Could you check a few things on this model? Use its own coordinates, in mm. Face numbers are marked on the shaded views. A direction names the side the tool comes from. Round coordinates to 2 decimals unless told otherwise and drop trailing zeros. Order: outer loops, then holes, each group sorted by start corner. A loop starts at its lowest first (then second) coordinate and runs counter-clockwise, first axis right, second up. Notation, with made-up numbers: (-25, 56) - (21, 56) arc R26 ccw to (21, 77) - close; hole circle Ø8 at (40, 44.5). An arc over 180 degrees is marked (long way). Return JSON: item names as keys, results as strings. Group by question number.
Autodesk Inventor part; units mm, degrees
ref_plane "Work Plane1" through (-3, -25.1, -19.1) normal (0, 0, 1) x (1, 0, 0)
ref_plane "YZ Plane" through (0, 0, 0) normal (1, 0, 0) x (0, 1, 0)
ref_plane "XZ Plane" through (0, 0, 0) normal (0, 1, 0) x (-1, 0, 0)
sketch "Sketch1" plane through (0, 0, 0) normal (1, 0, 0) x (0, 1, 0)
  line L0 (0, 0) -> (-25.1, 0)
  line L1 (-25.1, 0) -> (-25.1, -38.2)
  line L2 (-25.1, -38.2) -> (0, -38.2)
  line L3 (0, -38.2) -> (0, 0)
  circle A0 centre (-22.1, -15.85) radius 2.5
  circle A1 centre (-22.1, -22.35) radius 2.5
  arc A2 (-18.1, -15.85) -> (-25.1, -18.4958) centre (-22.1, -15.85) ccw
  arc A3 (-25.1, -19.7042) -> (-18.1, -22.35) centre (-22.1, -22.35) ccw
  line L4 (-18.1, -15.85) -> (-18.1, -22.35)
  line L5 (-22.1, -11.85) -> (-25.1, -11.85)
  line L6 (-22.1, -26.35) -> (-25.1, -26.35)
  line L7 (0, 0) -> (-25.1, 0)
  line L8 (-25.1, 0) -> (-25.1, 5)
  line L9 (-25.1, 5) -> (0, 5)
  line L10 (0, 5) -> (0, 0)
  line L11 (0, -38.2) -> (-25.1, -38.2)
  line L12 (-25.1, -38.2) -> (-25.1, -43.2)
  line L13 (-25.1, -43.2) -> (0, -43.2)
  line L14 (0, -43.2) -> (0, -38.2)
  point P0 (-25.1, -19.1)
  point P1 (-25.1, -13.2042)
  point P2 (-25.1, -24.9958)
  dimension "d0" = 38.2
  dimension "d1" = 25.1
  dimension "d2" = 5
  dimension "d3" = 6.5
  dimension "d4" = 3
  dimension "d5" = 3.25
  dimension "d6" = 8
  dimension "d11" = 5
  dimension "d12" = 5
extrude "Extrusion1" add sketch "Sketch1" against normal blind 3 contours L3 L2 L1 L6 A3 L4 A2 L5 L0 | L0 L8 L9 L10 | L14 L13 L12 L2 | L5 A2 L1 | A2 L4 A3 L1 | L1 A3 L6 | A0 | A1
extrude "Extrusion2" add sketch "Sketch1" along normal blind 11 contours L0 L8 L9 L10 | L14 L13 L12 L2 | L5 A2 L1 | A2 L4 A3 L1 | L1 A3 L6
sketch "Sketch2" plane through (-3, -25.1, 5) normal (0, 0, 1) x (1, 0, 0)
  circle A0 centre (7, 20.1) radius 2.6
  line L0 (0, 25.1) -> (14, 25.1)
  circle A1 centre (7, 8.1) radius 2.6
  point P0 (3, 25.1)
  point P1 (7, 25.1)
  dimension "d13" = 5.2
  dimension "d14" = 5
  dimension "d15" = 12
extrude "Extrusion3" [suppressed]
ref_plane "Work Plane1" through (-3, -25.1, -19.1) normal (0, 0, 1) x (1, 0, 0)
sketch "Sketch3" plane through (-3, 0, 5) normal (0, 1, 0) x (1, 0, 0)
  line L0 (14, 48.2) -> (0, 48.2)
  line L1 (0, 0) -> (0, 48.2)
  line L2 (0, 0) -> (14, 0)
  line L3 (14, 5) -> (14, 0)
  line L4 (3, 5) -> (14, 5)
  line L5 (3, 43.2) -> (3, 5)
  line L6 (3, 43.2) -> (14, 43.2)
  line L7 (14, 48.2) -> (14, 43.2)
  arc A0 (10.9206, 1.625) -> (6.0794, 1.625) centre (8.5, 1) ccw
  line L8 (10, 0.5) -> (10, 0)
  line L9 (7, 0.5) -> (7, 0)
  arc A1 (7, 0.5) -> (6.5, 1) centre (6.5, 0.5) ccw
  arc A2 (10.5, 1) -> (10, 0.5) centre (10.5, 0.5) ccw
  line L10 (6.5, 1) -> (6, 1)
  arc A3 (11, 1) -> (6, 1) centre (8.5, 1) ccw
  line L11 (10.5, 1) -> (11, 1)
  point P0 (8.5, 5)
  point P1 (7, 1)
  point P2 (10, 1)
  point P3 (10.9206, 1.625)
  point P4 (6.0794, 1.625)
  dimension "d23" = 5
  dimension "d26" = 1.5
  dimension "d28" = 1.5
  dimension "d31" = 0.5
extrude "Extrusion4" cut sketch "Sketch3" against normal through all contours L9 A1 L10 A3 A0 L11 A2 L8 L2
fillet "Fillet1" radius 0.5 2 edges at (3, -12.55, 4) (8, -12.55, 4)
properties part number "Pixy2 cover"
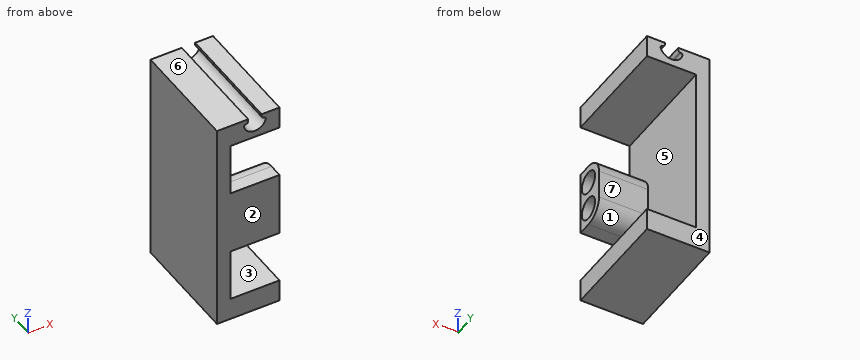
1) I want a section at B-B, the plane x = 4.75. List the corners of the cut face in (y, z) for me, plus the area to 3 significant figures.
2) For the marked faces 1, 2 and 3, which set-ups out of +Z, -Z, +X, -X, +Y, -Y let a thin tool reach every point of the face, with its end or its side?
3) We'd pull the mould along Z, two halves only. Please class the marked faces 4, 5, 6 and 7: +Z half, -Z half, draft (parallel to the pull), parting line (faces both ways), or undercut.
4) If I drill on line 1 along Z through (x, y) = (8.5, -12.25); line 2 along Z through (x, y) = (7.75, -10.75); line 3 along Z through (x, y) = (6, -22.1), over which ranges is the centre line in solid material (lowest first)? Write a range as from..to.
5) I want a section at D-D, the plane z = -3.5. List the corners of the cut face in (x, y) for me, plus the area to 3 significant figures.
6) I want a section at C-C, the plane z = -12.5. List the corners of the cut face in (x, y) for me, plus the area to 3 significant figures.
7) I want a section at A-A, the plane x = 2.25. List the corners of the cut face in (y, z) for me.
8) Will these pins go through, and if not, where does the flat tip stop? pin 1 (5.5 mm diameter, centred on y = -21, z = -17, fed in from +X); pin 2 (4.5 mm diameter, centred on y = -22.1, z = -15.85, fed in from +X); pin 3 (1 mm diameter, centred on x = 6, z = -36, fed in from +Y); pin 4 (6 mm diameter, centred on x = 9, z = -18, fed in from +Y).
Outcome:
{
 "1": {"outline": "(-25.1, -43.2) - (0, -43.2) - (0, -38.2) - (-25.1, -38.2) - close; (-25.1, -26.35) - (-22.1, -26.35) arc R4 ccw to (-18.1, -22.35) - (-18.1, -15.85) arc R4 ccw to (-22.1, -11.85) - (-25.1, -11.85) - close; (-25.1, 0) - (0, 0) - (0, 1.62) - (-25.1, 1.62) - close; hole circle Ø5 at (-22.1, -22.35); hole circle Ø5 at (-22.1, -15.85)", "area": "221 mm^2"},
 "2": {"face 1": "+X, +Y", "face 2": "+Z, -Z, +X, -X, -Y", "face 3": "+X, +Y, -Y"},
 "3": {"face 4": "draft", "face 5": "undercut", "face 6": "+Z half", "face 7": "undercut"},
 "4": {"line 1": "-43.2..-38.2, 0..5", "line 2": "-43.2..-38.2, 0..2.91, 3.89..5", "line 3": "-43.2..-38.2, -26.35..-24.85, -19.85..-18.35, -13.35..-11.85, 0..1.55"},
 "5": {"outline": "(-3, -25.1) - (0, -25.1) - (0, 0) - (-3, 0) - close", "area": "75.3 mm^2"},
 "6": {"outline": "(-3, -25.1) - (11, -25.1) - (11, -19.91) - (0, -19.91) - (0, 0) - (-3, 0) - close", "area": "132 mm^2"},
 "7": {"outline": "(-25.1, -43.2) - (0, -43.2) - (0, -38.2) - (-25.1, -38.2) - close; (-25.1, -26.35) - (-22.1, -26.35) arc R4 ccw to (-18.1, -22.35) - (-18.1, -15.85) arc R4 ccw to (-22.1, -11.85) - (-25.1, -11.85) - close; (-25.1, 0) - (0, 0) - (0, 5) - (-25.1, 5) - close; hole circle Ø5 at (-22.1, -22.35); hole circle Ø5 at (-22.1, -15.85)"},
 "8": {"pin 1": "x = 11", "pin 2": "x = 0", "pin 3": "through", "pin 4": "y = -18.1"}
}
